```python
from build123d import *

# Parameters (mm, degrees)
F0_R     = 15.25
F1_DEPTH = 1
F2_R     = 15.25
F2_R_2   = 14.6
F3_DEPTH = 3.25
F5_DEPTH = 4.251


with BuildPart() as f1:
    # F0 (on Top) → F1 (new body)
    with BuildSketch(Plane.XY):
        Circle(F0_R)
    extrude(amount=-F1_DEPTH)

    # F2 (on Top) → F3 (join)
    with BuildSketch(Plane.XY):
        Circle(F2_R)
        Circle(F2_R_2, mode=Mode.SUBTRACT)
        with BuildLine():
            ThreePointArc((1.4254005383, 4.426142034), (1.6960254298, 4.4160388114), (1.932222804, 4.5485178944))
            Line((1.932222804, 4.5485178944), (6.9650017947, 9.5812968851))
            ThreePointArc((6.9650017947, 9.5812968851), (7.0528697603, 9.7934289194), (6.9650017947, 10.0055609538))
            Line((6.9650017947, 10.0055609538), (6.8967918056, 10.0737709429))
            ThreePointArc((6.8967918056, 10.0737709429), (6.1879198942, 10.3666626039), (5.4800863823, 10.0712702695))
            Line((5.4800863823, 10.0712702695), (2.0984543523, 6.6656774564))
            ThreePointArc((2.0984543523, 6.6656774564), (1.6856522801, 6.4153428351), (1.2036749488, 6.3875790889))
            ThreePointArc((1.2036749488, 6.3875790889), (0.6044567486, 6.4718337462), (0, 6.5))
            ThreePointArc((0, 6.5), (-0.6044567486, 6.4718337462), (-1.2036749488, 6.3875790889))
            ThreePointArc((-1.2036749488, 6.3875790889), (-1.6856522801, 6.4153428351), (-2.0984543523, 6.6656774564))
            Line((-2.0984543523, 6.6656774564), (-5.4800863823, 10.0712702695))
            ThreePointArc((-5.4800863823, 10.0712702695), (-6.1879198942, 10.3666626039), (-6.8967918056, 10.0737709429))
            Line((-6.8967918056, 10.0737709429), (-6.9650017947, 10.0055609538))
            ThreePointArc((-6.9650017947, 10.0055609538), (-7.0528697603, 9.7934289194), (-6.9650017947, 9.5812968851))
            Line((-6.9650017947, 9.5812968851), (-1.932222804, 4.5485178944))
            ThreePointArc((-1.932222804, 4.5485178944), (-1.6960254298, 4.4160388114), (-1.4254005383, 4.426142034))
            ThreePointArc((-1.4254005383, 4.426142034), (-0.7214359091, 4.5936946164), (0, 4.65))
            ThreePointArc((0, 4.65), (0.7214359091, 4.5936946164), (1.4254005383, 4.426142034))
        make_face()
        with BuildLine():
            Line((10.0737709429, 6.8967918056), (10.0055609538, 6.9650017947))
            ThreePointArc((10.0055609538, 6.9650017947), (9.7934289194, 7.0528697603), (9.5812968851, 6.9650017947))
            Line((9.5812968851, 6.9650017947), (4.5485178944, 1.932222804))
            ThreePointArc((4.5485178944, 1.932222804), (4.4160388114, 1.6960254298), (4.426142034, 1.4254005383))
            ThreePointArc((4.426142034, 1.4254005383), (4.5936946164, 0.7214359091), (4.65, 0))
            ThreePointArc((4.65, 0), (4.5936946164, -0.7214359091), (4.426142034, -1.4254005383))
            ThreePointArc((4.426142034, -1.4254005383), (4.4160388114, -1.6960254298), (4.5485178944, -1.932222804))
            Line((4.5485178944, -1.932222804), (9.5812968851, -6.9650017947))
            ThreePointArc((9.5812968851, -6.9650017947), (9.7934289194, -7.0528697603), (10.0055609538, -6.9650017947))
            Line((10.0055609538, -6.9650017947), (10.0737709429, -6.8967918056))
            ThreePointArc((10.0737709429, -6.8967918056), (10.3666626039, -6.1879198942), (10.0712702695, -5.4800863823))
            Line((10.0712702695, -5.4800863823), (6.6656774564, -2.0984543523))
            ThreePointArc((6.6656774564, -2.0984543523), (6.4153428351, -1.6856522801), (6.3875790889, -1.2036749488))
            ThreePointArc((6.3875790889, -1.2036749488), (6.4718337462, -0.6044567486), (6.5, 0))
            ThreePointArc((6.5, 0), (6.4718337462, 0.6044567486), (6.3875790889, 1.2036749488))
            ThreePointArc((6.3875790889, 1.2036749488), (6.4153428351, 1.6856522801), (6.6656774564, 2.0984543523))
            Line((6.6656774564, 2.0984543523), (10.0712702695, 5.4800863823))
            ThreePointArc((10.0712702695, 5.4800863823), (10.3666626039, 6.1879198942), (10.0737709429, 6.8967918056))
        make_face()
        with BuildLine():
            ThreePointArc((-9.5812968851, 6.9650017947), (-9.7934289194, 7.0528697603), (-10.0055609538, 6.9650017947))
            Line((-10.0055609538, 6.9650017947), (-10.0737709429, 6.8967918056))
            ThreePointArc((-10.0737709429, 6.8967918056), (-10.3666626039, 6.1879198942), (-10.0712702695, 5.4800863823))
            Line((-10.0712702695, 5.4800863823), (-6.6656774564, 2.0984543523))
            ThreePointArc((-6.6656774564, 2.0984543523), (-6.4153428351, 1.6856522801), (-6.3875790889, 1.2036749488))
            ThreePointArc((-6.3875790889, 1.2036749488), (-6.4718337462, 0.6044567486), (-6.5, 0))
            ThreePointArc((-6.5, 0), (-6.4718337462, -0.6044567486), (-6.3875790889, -1.2036749488))
            ThreePointArc((-6.3875790889, -1.2036749488), (-6.4153428351, -1.6856522801), (-6.6656774564, -2.0984543523))
            Line((-6.6656774564, -2.0984543523), (-10.0712702695, -5.4800863823))
            ThreePointArc((-10.0712702695, -5.4800863823), (-10.3666626039, -6.1879198942), (-10.0737709429, -6.8967918056))
            Line((-10.0737709429, -6.8967918056), (-10.0055609538, -6.9650017947))
            ThreePointArc((-10.0055609538, -6.9650017947), (-9.7934289194, -7.0528697603), (-9.5812968851, -6.9650017947))
            Line((-9.5812968851, -6.9650017947), (-4.5485178944, -1.932222804))
            ThreePointArc((-4.5485178944, -1.932222804), (-4.4160388114, -1.6960254298), (-4.426142034, -1.4254005383))
            ThreePointArc((-4.426142034, -1.4254005383), (-4.5936946164, -0.7214359091), (-4.65, 0))
            ThreePointArc((-4.65, 0), (-4.5936946164, 0.7214359091), (-4.426142034, 1.4254005383))
            ThreePointArc((-4.426142034, 1.4254005383), (-4.4160388114, 1.6960254298), (-4.5485178944, 1.932222804))
            Line((-4.5485178944, 1.932222804), (-9.5812968851, 6.9650017947))
        make_face()
        with BuildLine():
            ThreePointArc((-6.9650017947, -9.5812968851), (-7.0528697603, -9.7934289194), (-6.9650017947, -10.0055609538))
            Line((-6.9650017947, -10.0055609538), (-6.8967918056, -10.0737709429))
            ThreePointArc((-6.8967918056, -10.0737709429), (-6.1879198942, -10.3666626039), (-5.4800863823, -10.0712702695))
            Line((-5.4800863823, -10.0712702695), (-2.0984543523, -6.6656774564))
            ThreePointArc((-2.0984543523, -6.6656774564), (-1.6856522801, -6.4153428351), (-1.2036749488, -6.3875790889))
            ThreePointArc((-1.2036749488, -6.3875790889), (-0.6044567486, -6.4718337462), (0, -6.5))
            ThreePointArc((0, -6.5), (0.6044567486, -6.4718337462), (1.2036749488, -6.3875790889))
            ThreePointArc((1.2036749488, -6.3875790889), (1.6856522801, -6.4153428351), (2.0984543523, -6.6656774564))
            Line((2.0984543523, -6.6656774564), (5.4800863823, -10.0712702695))
            ThreePointArc((5.4800863823, -10.0712702695), (6.1879198942, -10.3666626039), (6.8967918056, -10.0737709429))
            Line((6.8967918056, -10.0737709429), (6.9650017947, -10.0055609538))
            ThreePointArc((6.9650017947, -10.0055609538), (7.0528697603, -9.7934289194), (6.9650017947, -9.5812968851))
            Line((6.9650017947, -9.5812968851), (1.932222804, -4.5485178944))
            ThreePointArc((1.932222804, -4.5485178944), (1.6960254298, -4.4160388114), (1.4254005383, -4.426142034))
            ThreePointArc((1.4254005383, -4.426142034), (0.7214359091, -4.5936946164), (0, -4.65))
            ThreePointArc((0, -4.65), (-0.7214359091, -4.5936946164), (-1.4254005383, -4.426142034))
            ThreePointArc((-1.4254005383, -4.426142034), (-1.6960254298, -4.4160388114), (-1.932222804, -4.5485178944))
            Line((-1.932222804, -4.5485178944), (-6.9650017947, -9.5812968851))
        make_face()
    extrude(amount=F3_DEPTH)

    # F4 (on face) → F5 (cut, through all)
    with BuildSketch(Plane(origin=(0, 0, -1), x_dir=(1, 0, 0), z_dir=(0, 0, -1))):
        with BuildLine():
            Line((-2.1, 16), (-2.1, 1.3564659966))
            ThreePointArc((-2.1, 1.3564659966), (0, -2.5), (2.1, 1.3564659966))
            Line((2.1, 1.3564659966), (2.1, 16))
            Line((2.1, 16), (0, 16))
            Line((0, 16), (-2.1, 16))
        make_face()
    extrude(amount=-F5_DEPTH, mode=Mode.SUBTRACT)


solid = f1.part
```
Design review of the part built by this model. Coordinates are the model's own, in mm. A direction names the side the tool comes from. Give positions to 0.01 mm unless a question says otherwise; leave off trailing zeros. Write each loop counter-clockwise with the first axis right and the second up, starting at its lowest first coordinate (ties: lowest second). Pieces come first, ordered by that corner, then holes.
(1) Add section C-C (x = 12). Give the boundary of the cut face in (y, z).
Checked values:
outline: (-9.41, -1) - (9.41, -1) - (9.41, 3.25) - (8.32, 3.25) - (8.32, 0) - (-8.32, 0) - (-8.32, 3.25) - (-9.41, 3.25) - close
(2) Add section D-D (z = -0.5). Give the boundary of the cut face in (x, y), and give its area (3 significant figures).
Checked values:
outline: (-2.1, -15.1) - (-2.1, -1.36) arc R2.5 cw (long way) to (2.1, -1.36) - (2.1, -15.1) arc R15.25 ccw (long way) to start
area: 656 mm2
(3) Wall thickness on line 1 along Y through (x, z) = (8, 0.15); line 2 along Y through (x, z) = (5.5, 1.15); line 3 along X through (y, z) = (-5.5, 1.9): over which ranges is each line inside the solid? List them lowest first.
Checked values:
line 1: y = -12.98 to -12.21, -5.38 to -3.42, 3.42 to 5.38, 12.21 to 12.98
line 2: y = -14.22 to -13.52, -10.09 to -8.12, -2.88 to 2.88, 8.12 to 10.09, 13.52 to 14.22
line 3: x = -14.22 to -13.52, -10.09 to -8.12, -2.88 to -2.1, 2.1 to 2.88, 8.12 to 10.09, 13.52 to 14.22
(4) Clearance check with flat-ended pins moving along their axes: pin 1 Ø8.5 at (x, y) = (-6.5, -5) entering from +Z; pin 2 Ø1.5 at (x, z) = (3.5, 2.5) entering from -Y; pin 3 Ø1 at (x, y) = (-1, 1) entering from -Z; pin 4 Ø1.3 at (y, z) = (-10, 1) entering from -X. State where each tip first meets the part, or that it passes through.
Checked values:
pin 1: stops at z = 3.25
pin 2: stops at y = -15
pin 3: passes through
pin 4: stops at x = -12.05
(5) Mouldability with a two-part tool opening along X and no side actions: class faces 3 (the face through (-6.413, -1.679, 1.602)), 4 (the face through (-6, 0, 3.25)) as +X half, -X half, draft (parallel to the pull), parting line (faces both ways), or undercut.
Checked values:
face 3: undercut
face 4: draft
(6) Add section B-B (y = -4). Give the boundary of the cut face in (x, z).
Checked values:
outline: (-14.72, -1) - (-2.1, -1) - (-2.1, 0) - (-6.62, 0) - (-6.62, 3.25) - (-8.58, 3.25) - (-8.58, 0) - (-14.04, 0) - (-14.04, 3.25) - (-14.72, 3.25) - close; (2.1, -1) - (14.72, -1) - (14.72, 3.25) - (14.04, 3.25) - (14.04, 0) - (8.58, 0) - (8.58, 3.25) - (6.62, 3.25) - (6.62, 0) - (2.1, 0) - close
(7) Tool access review of faces 1 (the face through (-6.199, -10.367, 1.602)), 2 (the face through (3, 0, -1)): name each direction out of +Z, -Z, +X, -X, +Y, -Y from which nothing blocks a thin tool from reaching the whole face with its end or side.
Checked values:
face 1: +Z
face 2: -Z, +X, -X, +Y, -Y
(8) Add section A-A (z = 1.45). Give the number of separate pieces and of enclosed holes in the cut face, and give its area (3 significant figures).
Checked values:
separate pieces: 6
enclosed holes: 0
area: 152 mm2
